```python
from build123d import *

# Parameters (mm, degrees)
CYLINDER010_R                = 2.5
CYLINDER010_DEPTH            = 12
FUSION001018_PLACEMENT_ANGLE = 180


with BuildPart() as cone002:
    # Cone002 → Cone002 (revolve)
    with BuildSketch(Plane(origin=(0, 0, -3), x_dir=(1, 0, 0), z_dir=(0, -1, 0))):
        Polygon((0, 0), (4.5, 0), (2.5, 3), (0, 3), align=None)
    revolve(axis=Axis((0, 0, -3), (0, 0, 1)))


with BuildPart() as obj1:
    # Cylinder010 → Cylinder010 (new body)
    with BuildSketch(Plane.XY):
        Circle(CYLINDER010_R)
    extrude(amount=CYLINDER010_DEPTH)

    # Fusion001018: union Cone002
    add(cone002.part)


with BuildPart() as obj1_1:
    # Fusion001018 placement: moved
    add(obj1.part.moved(Location((45, 15, 21))).rotate(Axis((45, 15, 21), (0, 1, 0)), FUSION001018_PLACEMENT_ANGLE))


solid = obj1_1.part
```
Design review of the part built by this model. Coordinates are the model's own, in mm. A direction names the side the tool comes from. Give positions to 0.01 mm unless a question says otherwise; leave off trailing zeros. Write each loop counter-clockwise with the first axis right and the second up, starting at its lowest first coordinate (ties: lowest second). Pieces come first, ordered by that corner, then holes.
(1) Add section C-C (z = 12.75). Give the boundary of the cut face in (x, y).
Checked values:
outline: circle Ø5 at (45, 15)
(2) Clearance check with flat-ended pins moving along their axes: pin 1 Ø1.5 at (y, z) = (12, 13.5) entering from -X; pin 2 Ø1.5 at (y, z) = (16, 11.5) entering from +X; pin 3 Ø1.5 at (y, z) = (12.5, 21.5) entering from -X. State where each tip first meets the part, or that it passes through.
Checked values:
pin 1: stops at x = 43.91
pin 2: stops at x = 47.49
pin 3: stops at x = 42.49
(3) Add section D-D (z = 23.25). Give the boundary of the cut face in (x, y), and give its area (3 significant figures).
Checked values:
outline: circle Ø8 at (45, 15)
area: 50.3 mm2
(4) Wall thickness on line 1 along Z through (x, y) = (48.25, 12.75); line 2 along X through (y, z) = (13.25, 20.5); line 3 along Y through (x, z) = (46.5, 16): over which ranges is each line inside the solid? List them lowest first.
Checked values:
line 1: z = 23.18 to 24
line 2: x = 43.21 to 46.79
line 3: y = 13 to 17
(5) Add section B-B (y = 15). Give the boundary of the cut face in (x, z), and give its area (3 significant figures).
Checked values:
outline: (40.5, 24) - (42.5, 21) - (42.5, 9) - (47.5, 9) - (47.5, 21) - (49.5, 24) - close
area: 81.0 mm2
(6) Tool access review of faces 1 (the face through (42.69, 14.04, 15.08)), 2 (the face through (45, 15, 9)): name each direction out of +Z, -Z, +X, -X, +Y, -Y from which nothing blocks a thin tool from reaching the whole face with its end or side.
Checked values:
face 1: -Z
face 2: -Z, +X, -X, +Y, -Y
(7) Add section A-A (x = 45). Give the boundary of the cut face in (y, z).
Checked values:
outline: (10.5, 24) - (12.5, 21) - (12.5, 9) - (17.5, 9) - (17.5, 21) - (19.5, 24) - close
